```python
from build123d import *

# Parameters (mm, degrees)
F0_R     = 1.5
F1_DEPTH = 10
F2_R     = 3
F2_R_2   = 1.5
F3_DEPTH = 3
F4_R     = 1.5
F5_DEPTH = 2


with BuildPart() as f1:
    # F0 (on Front) → F1 (new body)
    with BuildSketch(Plane.XZ):
        Circle(F0_R)
    extrude(amount=-F1_DEPTH)

    # F2 (on face) → F3 (join)
    with BuildSketch(Plane.XZ):
        Circle(F2_R)
        Polygon((1.375, 2.3815698604), (2.75, 0), (1.375, -2.3815698604), (-1.375, -2.3815698604), (-2.75, 0), (-1.375, 2.3815698604), align=None, mode=Mode.SUBTRACT)
        Polygon((1.375, -2.3815698604), (2.75, 0), (1.375, 2.3815698604), (-1.375, 2.3815698604), (-2.75, 0), (-1.375, -2.3815698604), align=None)
        Circle(F2_R_2, mode=Mode.SUBTRACT)
    extrude(amount=-F3_DEPTH)

    # F4 (on face) → F5 (cut)
    with BuildSketch(Plane.XZ):
        Polygon((-1.5155444566, -0.875), (0, -1.75), (1.5155444566, -0.875), (1.5155444566, 0.875), (0, 1.75), (-1.5155444566, 0.875), align=None)
        Circle(F4_R, mode=Mode.SUBTRACT)
        Circle(F4_R)
    extrude(amount=-F5_DEPTH, mode=Mode.SUBTRACT)


solid = f1.part
```
Input: part model. Units: mm. Frame: model coordinates. A direction names the side the tool comes from. Give positions to 0.01 mm unless a question says otherwise; leave off trailing zeros. Order: outer loops, then holes, each group sorted by start corner. A loop starts at its lowest first (then second) coordinate and runs counter-clockwise, first axis right, second up.
1. Cut plane D-D (x = 2.25). Return loops of the section in (y, z), and give its area (3 significant figures).
Computed:
outline: (0, -1.98) - (3, -1.98) - (3, 1.98) - (0, 1.98) - close
area: 11.9 mm2
2. Set-up query: faces 4 (the face through (-0.747, 0.986, 1.319)), 5 (the face through (-3, 1, 0)), 6 (the face through (1.3, 3, -1.3)). Return all of +Z, -Z, +X, -X, +Y, -Y with unobstructed straight access to the full face (end or side cutting, diameter ignored); none if empty.
Computed:
face 4: -Y
face 5: +Y, -Y
face 6: +Y
3. Cut plane B-B (x = -1.25). Return loops of the section in (y, z).
Computed:
outline: (0, -2.73) - (3, -2.73) - (3, -0.83) - (10, -0.83) - (10, 0.83) - (3, 0.83) - (3, 2.73) - (0, 2.73) - (0, 1.03) - (2, 1.03) - (2, -1.03) - (0, -1.03) - close
4. Pin query (flat end, axial travel): pin 1 Ø2 at (x, y) = (1, 6) entering from +Z; pin 2 Ø0.5 at (y, z) = (0.5, -0.5) entering from -X; pin 3 Ø0.9 at (x, z) = (-0.5, -0.5) entering from -Y. Return the tip coordinate at first contact, or that it passes through.
Computed:
pin 1: stops at z = 1.5
pin 2: stops at x = -2.99
pin 3: stops at y = 2
5. Cut plane C-C (y = 6.5). Return loops of the section in (x, z).
Computed:
outline: circle Ø3 at (0, 0)
6. Draft query along Z for faces 1 (the face through (-1.5, 6.45, 0.07)), 2 (the face through (-0.768, 0.986, -1.306)), 3 (the face through (0, 10, 0)). Return one class per face: released by +Z, released by -Z, zero draft, split by the parting line, or undercut.
Computed:
face 1: split by the parting line
face 2: undercut
face 3: zero draft
7. Line query: probe 1 along Y at (x, z) = (-0.55, 0.05); probe 2 along X at (y, z) = (0.5, -1.3); probe 3 along Z at (x, y) = (-0.1, 1). Output: solid intervals per line, ascending.
Computed:
probe 1: y = 2 to 10
probe 2: x = -2.7 to -0.78, 0.78 to 2.7
probe 3: z = -3 to -1.69, 1.69 to 3
8. Cut plane A-A (z = 0). Return loops of the section in (x, y).
Computed:
outline: (-3, 0) - (-1.52, 0) - (-1.52, 2) - (1.52, 2) - (1.52, 0) - (3, 0) - (3, 3) - (1.5, 3) - (1.5, 10) - (-1.5, 10) - (-1.5, 3) - (-3, 3) - close
